Check sheet for the modelled part. Datum: model origin and axes. Units: mm. Give positions to 0.01 mm unless a question says otherwise; leave off trailing zeros. Order: outer loops, then holes, each group sorted by start corner. A loop starts at its lowest first (then second) coordinate and runs counter-clockwise, first axis right, second up.
from build123d import *

# Parameters (mm, degrees)
SKETCH_1_R               = 8
SKETCH_1_R_2             = 2
SKETCH_1_R_3             = 4
SKETCH_1_R_4             = 1.5
EXTRUDE_1_DEPTH          = 2
HOLE_WIZARD_1_AT_2_COUNT = 2
HOLE_WIZARD_1_AT_2_PITCH = 10
HOLE_WIZARD_1_AT_3_COUNT = 2
HOLE_WIZARD_1_AT_3_PITCH = 50.5
HOLE_WIZARD_1_AT_4_COUNT = 2
HOLE_WIZARD_1_AT_4_PITCH = 49.5


with BuildPart() as part:
    # 草图1 → 凸台-拉伸1 (new body)
    with BuildSketch(Plane.XY):
        with BuildLine():
            Line((-23.162071109, -54.533023266), (23.162071109, -54.533023266))
            ThreePointArc((23.162071109, -54.533023266), (29.234653864, -52.01767713), (31.75, -45.945094375))
            Line((31.75, -45.945094375), (31.75, 60.379047844))
            ThreePointArc((31.75, 60.379047844), (29.234653864, 66.451630598), (23.162071109, 68.966976734))
            Line((23.162071109, 68.966976734), (-23.162071109, 68.966976734))
            ThreePointArc((-23.162071109, 68.966976734), (-29.234653864, 66.451630598), (-31.75, 60.379047844))
            Line((-31.75, 60.379047844), (-31.75, -45.945094375))
            ThreePointArc((-31.75, -45.945094375), (-29.234653864, -52.01767713), (-23.162071109, -54.533023266))
        make_face()
        with Locations((-12.5, 50.466976734)):
            Circle(SKETCH_1_R, mode=Mode.SUBTRACT)
        with Locations((12.5, 50.466976734)):
            Circle(SKETCH_1_R, mode=Mode.SUBTRACT)
        with Locations((-12.749904554, -35.463254167)):
            Circle(SKETCH_1_R, mode=Mode.SUBTRACT)
        with Locations((12.75, -35.533023266)):
            Circle(SKETCH_1_R, mode=Mode.SUBTRACT)
        with Locations((12.75, -10.033023266)):
            Circle(SKETCH_1_R, mode=Mode.SUBTRACT)
        with Locations((-12.749904554, -9.963254167)):
            Circle(SKETCH_1_R, mode=Mode.SUBTRACT)
        with Locations((24.75, 28.466976734)):
            Circle(SKETCH_1_R_2, mode=Mode.SUBTRACT)
        with Locations((24.75, 18.466976734)):
            Circle(SKETCH_1_R_2, mode=Mode.SUBTRACT)
        with Locations((-24.75, 28.466976734)):
            Circle(SKETCH_1_R_2, mode=Mode.SUBTRACT)
        with Locations((-24.75, 18.466976734)):
            Circle(SKETCH_1_R_2, mode=Mode.SUBTRACT)
        with Locations((0, 30.466976734)):
            Circle(SKETCH_1_R_3, mode=Mode.SUBTRACT)
        with Locations((-10.5, 18.466976734)):
            Circle(SKETCH_1_R_3, mode=Mode.SUBTRACT)
        with Locations((10.5, 18.466976734)):
            Circle(SKETCH_1_R_3, mode=Mode.SUBTRACT)
        with Locations((10.5, 25.466976734)):
            Circle(SKETCH_1_R_4, mode=Mode.SUBTRACT)
        with Locations((0, 37.466976734)):
            Circle(SKETCH_1_R_4, mode=Mode.SUBTRACT)
        with Locations((7, 30.466976734)):
            Circle(SKETCH_1_R_4, mode=Mode.SUBTRACT)
        with Locations((-10.5, 25.466976734)):
            Circle(SKETCH_1_R_4, mode=Mode.SUBTRACT)
        with Locations((0, 23.466976734)):
            Circle(SKETCH_1_R_4, mode=Mode.SUBTRACT)
        with Locations((-7, 30.466976734)):
            Circle(SKETCH_1_R_4, mode=Mode.SUBTRACT)
        with Locations((17.5, 18.466976734)):
            Circle(SKETCH_1_R_4, mode=Mode.SUBTRACT)
        with Locations((10.5, 11.466976734)):
            Circle(SKETCH_1_R_4, mode=Mode.SUBTRACT)
        with Locations((3.5, 18.466976734)):
            Circle(SKETCH_1_R_4, mode=Mode.SUBTRACT)
        with Locations((-3.5, 18.466976734)):
            Circle(SKETCH_1_R_4, mode=Mode.SUBTRACT)
        with Locations((-10.5, 11.466976734)):
            Circle(SKETCH_1_R_4, mode=Mode.SUBTRACT)
        with Locations((-17.5, 18.466976734)):
            Circle(SKETCH_1_R_4, mode=Mode.SUBTRACT)
    extrude(amount=EXTRUDE_1_DEPTH)

    # 草图4 → 打孔尺寸开槽半沉头螺钉的类型1 (revolve, cut)
    with BuildSketch(Plane(origin=(24.75, 28.466976734, 0), x_dir=(0, 1, 0), z_dir=(1, 0, 0))):
        Polygon((0, 0), (0, 3.021463052), (1.7, 2), (1.7, 1.5), (3.2, 0), align=None)
    hole_wizard_1 = revolve(axis=Axis((24.75, 28.466976734, -6.35), (0, 0, 1)), mode=Mode.SUBTRACT)

    # 打孔尺寸开槽半沉头螺钉的类型1 at 2: 打孔尺寸开槽半沉头螺钉的类型1 ×2
    with Locations(*[(0, -i * HOLE_WIZARD_1_AT_2_PITCH, 0) for i in range(1, HOLE_WIZARD_1_AT_2_COUNT)]):
        add(hole_wizard_1, mode=Mode.SUBTRACT)

    # 打孔尺寸开槽半沉头螺钉的类型1 at 3: 打孔尺寸开槽半沉头螺钉的类型1 ×2
    with Locations(*[Vector(-0.9801980198019802, -0.19801980198019808, 0) * (i * HOLE_WIZARD_1_AT_3_PITCH) for i in range(1, HOLE_WIZARD_1_AT_3_COUNT)]):
        add(hole_wizard_1, mode=Mode.SUBTRACT)

    # 打孔尺寸开槽半沉头螺钉的类型1 at 4: 打孔尺寸开槽半沉头螺钉的类型1 ×2
    with Locations(*[(-i * HOLE_WIZARD_1_AT_4_PITCH, 0, 0) for i in range(1, HOLE_WIZARD_1_AT_4_COUNT)]):
        add(hole_wizard_1, mode=Mode.SUBTRACT)


solid = part.part
1) Section check B-B, the plane x = 24.75. Record the cut outline in (y, z).
Recorded:
outline: (-54.38, 0) - (15.27, 0) - (16.47, 1.2) - (16.47, 2) - (-54.38, 2) - close; (20.47, 1.2) - (21.67, 0) - (25.27, 0) - (26.47, 1.2) - (26.47, 2) - (20.47, 2) - close; (30.47, 1.2) - (31.67, 0) - (68.82, 0) - (68.82, 2) - (30.47, 2) - close
2) Section check C-C, the plane z = 0.35. State how many separate pieces and enclosed holes the cut face has, then the cut area to 3 significant figures.
Recorded:
separate pieces: 1
enclosed holes: 25
area: 6,230 mm2
3) Depth check by flat-ended pin: pin 1 Ø4 at (x, y) = (-19.5, 7) entering from -Z; pin 2 Ø1.8 at (x, y) = (-7, 30.47) entering from -Z. Enter the tip coordinate at first touch or a pass-through.
Recorded:
pin 1: stops at z = 0
pin 2: passes through
4) Draft check along X on faces 1 (the face through (0, 8, 0)), 2 (the face through (-8.5, 30.5, 1)), 3 (the face through (-29.168, 66.518, 0.986)). Enter one of: +X half, -X half, draft (parallel to the pull), parting line (faces both ways), or undercut.
Recorded:
face 1: draft
face 2: undercut
face 3: -X half
5) Material ranges on L1, parallel to Y at x = 0, z = 0.55; L2, parallel to X at y = -10.5, z = 1.4; L3, parallel to Y at x = -0.5, z = 1.6, recorded low to high.
Recorded:
L1: y = -54.53 to 21.97, 24.97 to 26.47, 34.47 to 35.97, 38.97 to 68.97
L2: x = -31.75 to -20.73, -4.77 to 4.76, 20.74 to 31.75
L3: y = -54.53 to 22.05, 24.88 to 26.5, 34.44 to 36.05, 38.88 to 68.97
6) Section check D-D, the plane y = -33.5. Record the cut outline in (x, z), then the cut area to 3 significant figures.
Recorded:
outline: (-31.75, 0) - (-20.51, 0) - (-20.51, 2) - (-31.75, 2) - close; (-4.99, 0) - (5.01, 0) - (5.01, 2) - (-4.99, 2) - close; (20.49, 0) - (31.75, 0) - (31.75, 2) - (20.49, 2) - close
area: 65.0 mm2
7) Section check A-A, the plane x = 17.5. Record the cut outline in (y, z).
Recorded:
outline: (-54.53, 0) - (-41.97, 0) - (-41.97, 2) - (-54.53, 2) - close; (-29.1, 0) - (-16.47, 0) - (-16.47, 2) - (-29.1, 2) - close; (-3.6, 0) - (16.97, 0) - (16.97, 2) - (-3.6, 2) - close; (19.97, 0) - (44.22, 0) - (44.22, 2) - (19.97, 2) - close; (56.71, 0) - (68.97, 0) - (68.97, 2) - (56.71, 2) - close
